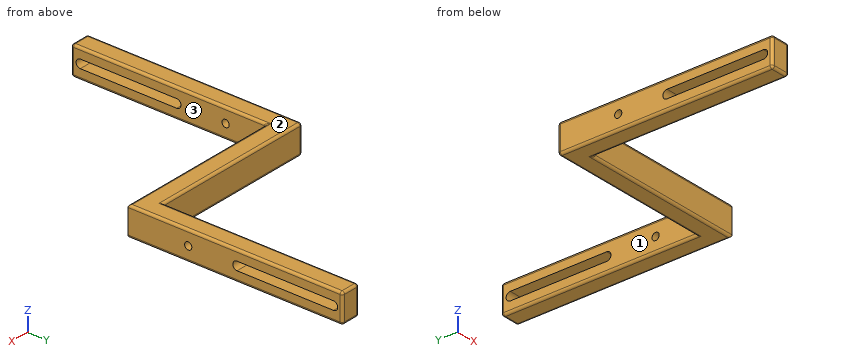
```python
from build123d import *

# Parameters (mm, degrees)
PAD_DEPTH       = 12
POCKET_DEPTH    = 8
SKETCH002_R     = 1.5
POCKET001_DEPTH = 8
SKETCH003_R     = 1.5
POCKET002_DEPTH = 8
FILLET_R        = 1
FILLET001_R     = 1
FILLET002_R     = 1
FILLET003_R     = 1
FILLET004_R     = 1
FILLET005_R     = 1
FILLET006_R     = 1
FILLET007_R     = 1


with BuildPart() as part:
    # Sketch → Pad (new body)
    with BuildSketch(Plane.XY):
        Polygon((8, 0), (0, 0), (0, 89), (68.5, 89), (68.5, 170), (76.5, 170), (76.5, 81), (8, 81), align=None)
    extrude(amount=PAD_DEPTH)

    # Sketch001 (on Face2 of Pad) → Pocket (cut)
    with BuildSketch(Plane(origin=(0, 0, 0), x_dir=(0, -1, 0), z_dir=(-1, 0, 0))):
        with BuildLine():
            ThreePointArc((-43.75, 7.75), (-45.5, 6), (-43.75, 4.25))
            Line((-43.75, 4.25), (-3.75, 4.25))
            ThreePointArc((-3.75, 4.25), (-2, 6), (-3.75, 7.75))
            Line((-3.75, 7.75), (-43.75, 7.75))
        make_face()
    extrude(amount=-POCKET_DEPTH, mode=Mode.SUBTRACT)

    # Sketch002 (on Face3 of Pocket) → Pocket001 (cut)
    with BuildSketch(Plane(origin=(0, 0, 0), x_dir=(0, -1, 0), z_dir=(-1, 0, 0))):
        with Locations((-64, 6)):
            Circle(SKETCH002_R)
    extrude(amount=-POCKET001_DEPTH, mode=Mode.SUBTRACT)

    # Sketch003 (on Face15 of Pocket001) → Pocket002 (cut)
    with BuildSketch(Plane.YZ.offset(76.5)):
        with Locations((106, 6)):
            Circle(SKETCH003_R)
        with BuildLine():
            ThreePointArc((126.25, 7.75), (124.5, 6), (126.25, 4.25))
            Line((126.25, 4.25), (166.25, 4.25))
            ThreePointArc((166.25, 4.25), (168, 6), (166.25, 7.75))
            Line((166.25, 7.75), (126.25, 7.75))
        make_face()
    extrude(amount=-POCKET002_DEPTH, mode=Mode.SUBTRACT)

    # Fillet
    fillet_edges = [part.edges().sort_by_distance(p)[0] for p in [
        (76.5, 125.5, 0),
        (42.25, 81, 0),
        (8, 40.5, 0),
        (8, 40.5, 12),
        (42.25, 81, 12),
        (76.5, 125.5, 12),
    ]]
    fillet(fillet_edges, radius=FILLET_R)

    # Fillet001
    fillet001_edges = [part.edges().sort_by_distance(p)[0] for p in [
        (68.5, 170, 6),
    ]]
    fillet(fillet001_edges, radius=FILLET001_R)

    # Fillet002
    fillet002_edges = [part.edges().sort_by_distance(p)[0] for p in [
        (68.5, 129, 12),
    ]]
    fillet(fillet002_edges, radius=FILLET002_R)

    # Fillet003
    fillet003_edges = [part.edges().sort_by_distance(p)[0] for p in [
        (34.25, 89, 0),
    ]]
    fillet(fillet003_edges, radius=FILLET003_R)

    # Fillet004
    fillet004_edges = [part.edges().sort_by_distance(p)[0] for p in [
        (34.25, 89, 12),
    ]]
    fillet(fillet004_edges, radius=FILLET004_R)

    # Fillet005
    fillet005_edges = [part.edges().sort_by_distance(p)[0] for p in [
        (0, 0, 6),
    ]]
    fillet(fillet005_edges, radius=FILLET005_R)

    # Fillet006
    fillet006_edges = [part.edges().sort_by_distance(p)[0] for p in [
        (0, 44.5, 12),
    ]]
    fillet(fillet006_edges, radius=FILLET006_R)

    # Fillet007
    fillet007_edges = [part.edges().sort_by_distance(p)[0] for p in [
        (8, 81, 6),
    ]]
    fillet(fillet007_edges, radius=FILLET007_R)


solid = part.part
```
Geometry check sheet. Reference: the model listing, model coordinates, mm. Face numbers are marked on the shaded views. A direction names the side the tool comes from. Give positions to 0.01 mm unless a question says otherwise; leave off trailing zeros. Write each loop counter-clockwise with the first axis right and the second up, starting at its lowest first coordinate (ties: lowest second). Pieces come first, ordered by that corner, then holes.
1) Gauge pin test, flat ends, axial feed: pin 1 (3.5 mm diameter, centred on y = 64, z = 6, fed in from -X); pin 2 (5 mm diameter, centred on x = 45, z = 8.5, fed in from +Y); pin 3 (5 mm diameter, centred on x = 37.5, z = 4.5, fed in from -Y). Record the tip position at first contact, or that the pin passes through.
2) Access from +Z, -Z, +X, -X, +Y, -Y to the whole of each face (thin tool, end or side, straight path). Record for the marked faces 1, 2 and 3.
3) Section check C-C, the plane x = 60.5. Record the boundary of the cut face in (y, z), and give its area (3 significant figures).
4) Material ranges on L1, parallel to Z at x = 3.5, y = 64; L2, parallel to Y at x = 55.5, z = 6.5; L3, parallel to X at y = 33, z = 2.75, recorded low to high.
5) Section check A-A, the plane y = 64. Record the boundary of the cut face in (x, z), and give its area (3 significant figures).
6) Section check D-D, the plane y = 155.5. Record the boundary of the cut face in (x, z).
7) Section check B-B, the plane y = 102.5. Record the boundary of the cut face in (x, z), and give its area (3 significant figures).
Computed:
1. pin 1: stops at x = 0
1. pin 2: stops at y = 89
1. pin 3: stops at y = 81
2. face 1: +Z, -Z, -X, +Y
2. face 2: +Z, +X, -X, +Y, -Y
2. face 3: +Z, -Z, +X, -Y
3. outline: (81, 1) arc R1 ccw to (82, 0) - (88, 0) arc R1 ccw to (89, 1) - (89, 11) arc R1 ccw to (88, 12) - (82, 12) arc R1 ccw to (81, 11) - close
3. area: 95.1 mm2
4. L1: z = 0 to 4.5, 7.5 to 12
4. L2: y = 81 to 89
4. L3: x = 0 to 8
5. outline: (0, 1) arc R1 ccw to (1, 0) - (7, 0) arc R1 ccw to (8, 1) - (8, 4.5) - (0, 4.5) - close; (0, 7.5) - (8, 7.5) - (8, 11) arc R1 ccw to (7, 12) - (1, 12) arc R1 ccw to (0, 11) - close
5. area: 71.1 mm2
6. outline: (68.5, 1) arc R1 ccw to (69.5, 0) - (75.5, 0) arc R1 ccw to (76.5, 1) - (76.5, 4.25) - (68.5, 4.25) - close; (68.5, 7.75) - (76.5, 7.75) - (76.5, 11) arc R1 ccw to (75.5, 12) - (69.5, 12) arc R1 ccw to (68.5, 11) - close
7. outline: (68.5, 1) arc R1 ccw to (69.5, 0) - (75.5, 0) arc R1 ccw to (76.5, 1) - (76.5, 11) arc R1 ccw to (75.5, 12) - (69.5, 12) arc R1 ccw to (68.5, 11) - close
7. area: 95.1 mm2
